Geometry: final body of the model. Coordinates: model frame, mm. A direction names the side the tool comes from. Give positions to 0.01 mm unless a question says otherwise; leave off trailing zeros. Write each loop counter-clockwise with the first axis right and the second up, starting at its lowest first coordinate (ties: lowest second). Pieces come first, ordered by that corner, then holes. Notation, with made-up numbers: (-33.75, -25) - (13.25, -25) arc R32 cw to (13.25, 3) - close; hole circle Ø10 at (3.5, 46.25). An arc over 180 degrees is marked (long way). Use CSV: the item, a comma, the result in double quotes. Start each with the question number.
(1) First-contact query: pin 1 Ø10 at (x, z) = (-3.5, 69.5) entering from -Y. Flat tip, straight axial feed; report the tip coordinate or a pass-through.
(2) Section C-C on x = 0. Output: boundary loops of the cut face in (y, z).
(3) Reachability of faces 1 (the flat face through (25.4, 0, 188)), 2 (the flat face through (0, -11.112, 188)), 3 (the cylindrical face through (1.599, 11.917, 61.916)) from +Z, -Z, +X, -X, +Y, -Y: full face, straight path, thin tool, end or side. Return the list, or none.
(4) Line query: probe 1 along Z at (x, y) = (0, -11.7); probe 2 along Y at (x, z) = (5, 38.5); probe 3 along X at (y, z) = (11.55, 355.6). Output: solid intervals per line, ascending. Write a range as [from, to].
(5) Draft query along Z for faces 4 (the flat face through (0, -12, 381)), 5 (the flat face through (0, -12, 0)), 6 (the cylindrical face through (5.47, 11.9, 368.8)), 7 (the flat face through (-25.4, 0, 188)). Return one class per face: released by +Z, released by -Z, zero draft, split by the parting line, or undercut.
(6) Section B-B on y = 4. Output: boundary loops of the cut face in (x, z).
(7) Section D-D on z = 355.6. Output: boundary loops of the cut face in (x, y).
(8) Section A-A on z = 302.5. Output: boundary loops of the cut face in (x, y), and give its area (3 significant figures).
Autodesk Inventor part; units mm, degrees
ref_plane "YZ Plane" through (0, 0, 0) normal (1, 0, 0) x (0, 1, 0)
ref_plane "XZ Plane" through (0, 0, 0) normal (0, 1, 0) x (-1, 0, 0)
ref_plane "XY Plane" through (0, 0, 0) normal (0, 0, 1) x (1, 0, 0)
sketch "Sketch1" plane through (0, 0, 0) normal (0, 0, 1) x (1, 0, 0)
  line L0 (-25.4, 12.7) -> (25.4, 12.7)
  line L1 (25.4, 12.7) -> (25.4, -12.7)
  line L2 (25.4, -12.7) -> (-25.4, -12.7)
  line L3 (-25.4, -12.7) -> (-25.4, 12.7)
  line L4 (-25.4, 12.7) -> (25.4, -12.7) construction
  line L5 (25.4, 12.7) -> (-25.4, -12.7) construction
  line L6 (-23.8125, 11.1125) -> (23.8125, 11.1125)
  line L7 (23.8125, 11.1125) -> (23.8125, -11.1125)
  line L8 (23.8125, -11.1125) -> (-23.8125, -11.1125)
  line L9 (-23.8125, -11.1125) -> (-23.8125, 11.1125)
  line L10 (-23.8125, 11.1125) -> (23.8125, -11.1125) construction
  line L11 (23.8125, 11.1125) -> (-23.8125, -11.1125) construction
  point P0 (0, 0)
  dimension "d0" = 50.8
  dimension "d1" = 25.4
  dimension "d2" = 47.625
  dimension "d3" = 22.225
extrude "Extrusion1" add sketch "Sketch1" along normal blind 381
sketch "Sketch2" plane through (-25.4, 12.7, 0) normal (0, 1, 0) x (1, 0, 0)
  line L0 (0, 0) -> (0, -381)
  line L1 (50.8, -381) -> (0, -381)
  point P0 (25.4, 0)
  point P1 (25.4, -355.6)
  dimension "d13" = 25.4
  dimension "d14" = 25.4
hole "Hole1" at (0, 12.7, 355.6) direction (0, -1, 0) diameter 28.575 end through all
sketch "Sketch3" plane through (-25.4, 12.7, 0) normal (0, 1, 0) x (1, 0, 0)
  line L0 (40.972, -76.2) -> (40.972, -141.2421)
  arc A0 (40.972, -76.2) -> (12.397, -76.2) centre (26.6845, -76.2) ccw
  line L1 (12.397, -141.2421) -> (12.397, -76.2)
  arc A1 (12.397, -141.2421) -> (40.972, -141.2421) centre (26.6845, -139.7) ccw
  line L2 (50.8, 0) -> (0, 0)
  line L3 (50.8, -381) -> (0, -381)
  circle A2 centre (25.4, -355.6) radius 14.2875
  point P0 (25.4, 0)
  dimension "d15" = 28.575
  dimension "d18" = 304.8
  dimension "d24" = 215.9
  dimension "d25" = 63.5
extrude "Extrusion2" cut sketch "Sketch3" against normal through all contours L0 A1 L1 A0
properties part number "Frame" material "Aluminum 6061"
Check values:
1,pin 1,"passes through"
2,outline,"(-12.7, 0) - (-11.11, 0) - (-11.11, 61.97) - (-12.7, 61.97) - close; (-12.7, 154.01) - (-11.11, 154.01) - (-11.11, 341.31) - (-12.7, 341.31) - close; (-12.7, 369.89) - (-11.11, 369.89) - (-11.11, 381) - (-12.7, 381) - close; (11.11, 0) - (12.7, 0) - (12.7, 61.97) - (11.11, 61.97) - close; (11.11, 154.01) - (12.7, 154.01) - (12.7, 341.31) - (11.11, 341.31) - close; (11.11, 369.89) - (12.7, 369.89) - (12.7, 381) - (11.11, 381) - close"
3,face 1,"+Z, -Z, +X, +Y, -Y"
3,face 2,"+Z, -Z"
3,face 3,"+Y, -Y"
4,probe 1,"z = [0, 61.97], [154.01, 341.31], [369.89, 381]"
4,probe 2,"y = [-12.7, -11.11], [11.11, 12.7]"
4,probe 3,"x = [-25.4, -14.29], [14.29, 25.4]"
5,face 4,"released by +Z"
5,face 5,"released by -Z"
5,face 6,"undercut"
5,face 7,"zero draft"
6,outline,"(-25.4, 0) - (-23.81, 0) - (-23.81, 381) - (-25.4, 381) - close; (23.81, 0) - (25.4, 0) - (25.4, 381) - (23.81, 381) - close"
7,outline,"(-25.4, -12.7) - (-14.29, -12.7) - (-14.29, -11.11) - (-23.81, -11.11) - (-23.81, 11.11) - (-14.29, 11.11) - (-14.29, 12.7) - (-25.4, 12.7) - close; (14.29, -12.7) - (25.4, -12.7) - (25.4, 12.7) - (14.29, 12.7) - (14.29, 11.11) - (23.81, 11.11) - (23.81, -11.11) - (14.29, -11.11) - close"
8,outline,"(-25.4, -12.7) - (25.4, -12.7) - (25.4, 12.7) - (-25.4, 12.7) - close; hole (-23.81, -11.11) - (23.81, -11.11) - (23.81, 11.11) - (-23.81, 11.11) - close"
8,area,"232 mm²"
